from build123d import *

# Parameters (mm, degrees)
SKETCH1_R              = 1.5
SKETCH1_W              = 20
SKETCH1_H              = 1.5
SKETCH1_W_2            = 22.82
SKETCH1_H_2            = 7.086
BOSS_EXTRUDE1_DEPTH    = 5
SKETCH1_3_W            = 22.82
SKETCH1_3_H            = 1.114
BOSS_EXTRUDE2_DEPTH    = 1
CUT_EXTRUDE1_DEPTH     = 23.696190187
LPATTERN1_COUNT        = 4
LPATTERN1_PITCH        = 5
BOSS_EXTRUDE3_START    = -12
SKETCH1_5_W            = 22.82
SKETCH1_5_H            = 7.086
SKETCH1_5_H_2          = 1.114
BOSS_EXTRUDE3_DEPTH    = 12
SKETCH4_W              = 0.5
SKETCH4_H              = 0.5
BOSS_EXTRUDE4_DEPTH    = 5
SKETCH5_W              = 0.5
SKETCH5_H              = 2
BOSS_EXTRUDE5_DEPTH    = 8
FILLET1_R              = 1
LPATTERN2_COUNT        = 4
LPATTERN2_PITCH        = 5
FILLET1_OF_LPATTERN2_R = 1


with BuildPart() as part:
    # Sketch1 → Boss-Extrude1 (new body)
    # profile 1 of 3: a face of its own
    with BuildSketch(Plane.XY):
        Polygon((20, 7.493), (-20, 7.493), (-20, -7.493), (-11.41, -7.493), (-11.41, -0.407), (11.41, -0.407), (11.41, -7.493), (20, -7.493), align=None)
        with Locations((-15.24, 2.993)):
            Circle(SKETCH1_R, mode=Mode.SUBTRACT)
        with Locations((0, 1.743)):
            Rectangle(SKETCH1_W, SKETCH1_H, mode=Mode.SUBTRACT)
        with Locations((15.24, 2.993)):
            Circle(SKETCH1_R, mode=Mode.SUBTRACT)
    # profile 2 of 3: a face of its own
    with BuildSketch(Plane.XY):
        with Locations((0, -3.95)):
            Rectangle(SKETCH1_W_2, SKETCH1_H_2)
        with BuildLine():
            Line((-10, -0.607), (-5, -0.607))
            Line((-5, -0.607), (-5, -6.007))
            Line((-5, -6.007), (-5.9, -6.007))
            ThreePointArc((-5.9, -6.007), (-7.5, -6.807), (-9.1, -6.007))
            Line((-9.1, -6.007), (-10, -6.007))
            Line((-10, -6.007), (-10, -0.607))
        make_face(mode=Mode.SUBTRACT)
    # profile 3 of 3: a face of its own
    with BuildSketch(Plane.XY):
        with BuildLine():
            Line((-10, -6.007), (-9.1, -6.007))
            ThreePointArc((-9.1, -6.007), (-7.5, -6.807), (-5.9, -6.007))
            Line((-5.9, -6.007), (-5, -6.007))
            Line((-5, -6.007), (-5, -0.607))
            Line((-5, -0.607), (-10, -0.607))
            Line((-10, -0.607), (-10, -6.007))
        make_face()
    extrude(amount=BOSS_EXTRUDE1_DEPTH)

    # Sketch1<3> → Boss-Extrude2 (add)
    with BuildSketch(Plane.XY):
        Polygon((-11.41, -7.493), (-20, -7.493), (-20, -9.493), (20, -9.493), (20, -7.493), (11.41, -7.493), (11.41, -8.607), (-11.41, -8.607), align=None)
        with Locations((0, -8.05)):
            Rectangle(SKETCH1_3_W, SKETCH1_3_H)
    extrude(amount=BOSS_EXTRUDE2_DEPTH)

    # Sketch1<4> → Cut-Extrude1 (cut, through all)
    with BuildSketch(Plane.XY):
        with BuildLine():
            Line((-10, -6.007), (-9.1, -6.007))
            ThreePointArc((-9.1, -6.007), (-7.5, -6.807), (-5.9, -6.007))
            Line((-5.9, -6.007), (-5, -6.007))
            Line((-5, -6.007), (-5, -0.607))
            Line((-5, -0.607), (-10, -0.607))
            Line((-10, -0.607), (-10, -6.007))
        make_face()
    cut_extrude1 = extrude(amount=CUT_EXTRUDE1_DEPTH, mode=Mode.SUBTRACT)

    # LPattern1: Cut-Extrude1 ×4
    with Locations(*[(i * LPATTERN1_PITCH, 0, 0) for i in range(1, LPATTERN1_COUNT)]):
        add(cut_extrude1, mode=Mode.SUBTRACT)

    # Sketch1<5> → Boss-Extrude3 (add)
    # profile 1 of 3: a face of its own
    with BuildSketch(Plane.XY.offset(BOSS_EXTRUDE3_START)):
        with Locations((0, -3.95)):
            Rectangle(SKETCH1_5_W, SKETCH1_5_H)
        with BuildLine():
            Line((-10, -0.607), (-5, -0.607))
            Line((-5, -0.607), (-5, -6.007))
            Line((-5, -6.007), (-5.9, -6.007))
            ThreePointArc((-5.9, -6.007), (-7.5, -6.807), (-9.1, -6.007))
            Line((-9.1, -6.007), (-10, -6.007))
            Line((-10, -6.007), (-10, -0.607))
        make_face(mode=Mode.SUBTRACT)
    # profile 2 of 3: a face of its own
    with BuildSketch(Plane.XY.offset(BOSS_EXTRUDE3_START)):
        with BuildLine():
            Line((-10, -6.007), (-9.1, -6.007))
            ThreePointArc((-9.1, -6.007), (-7.5, -6.807), (-5.9, -6.007))
            Line((-5.9, -6.007), (-5, -6.007))
            Line((-5, -6.007), (-5, -0.607))
            Line((-5, -0.607), (-10, -0.607))
            Line((-10, -0.607), (-10, -6.007))
        make_face()
    # profile 3 of 3: a face of its own
    with BuildSketch(Plane.XY.offset(BOSS_EXTRUDE3_START)):
        with Locations((0, -8.05)):
            Rectangle(SKETCH1_5_W, SKETCH1_5_H_2)
    extrude(amount=BOSS_EXTRUDE3_DEPTH)

    # Sketch4 → Boss-Extrude4 (add)
    with BuildSketch(Plane.XY):
        with Locations((-7.5, -3.307)):
            Rectangle(SKETCH4_W, SKETCH4_H)
    boss_extrude4 = extrude(amount=BOSS_EXTRUDE4_DEPTH)

    # Sketch5 → Boss-Extrude5 (add)
    with BuildSketch(Plane(origin=(0, 0, -12), x_dir=(-1, 0, 0), z_dir=(0, 0, -1))):
        with Locations((8.245, -4.507)):
            Rectangle(SKETCH5_W, SKETCH5_H)
    boss_extrude5 = extrude(amount=BOSS_EXTRUDE5_DEPTH)

    # Fillet1
    fillet1_edges = [part.edges().sort_by_distance(p)[0] for p in [
        (-8.245, -5.507, -20),
        (-8.245, -3.507, -20),
    ]]
    fillet(fillet1_edges, radius=FILLET1_R - 0.0001)  # a hair under: the kernel refuses the full size

    # LPattern2: Boss-Extrude4, Boss-Extrude5 ×4
    with Locations(*[(i * LPATTERN2_PITCH, 0, 0) for i in range(1, LPATTERN2_COUNT)]):
        add(boss_extrude4)
        add(boss_extrude5)

    # Fillet1 of LPattern2
    fillet1_of_lpattern2_edges = [part.edges().sort_by_distance(p)[0] for p in [
        (-3.245, -5.507, -20),
        (-3.245, -3.507, -20),
        (1.755, -5.507, -20),
        (1.755, -3.507, -20),
        (6.755, -5.507, -20),
        (6.755, -3.507, -20),
    ]]
    fillet(fillet1_of_lpattern2_edges, radius=FILLET1_OF_LPATTERN2_R - 0.0001)  # a hair under: the kernel refuses the full size


solid = part.part
CAD build for the part. Positions are in the model's coordinates, mm. A direction names the side the tool comes from. Coordinates: 2 decimals unless noted, no trailing zeros. Order: outer loops, then holes, each group sorted by start corner. A loop starts at its lowest first (then second) coordinate and runs counter-clockwise, first axis right, second up.
Item 1: Band-saw the part on B-B on x = 15.24. List the corners of the cut face in (y, z).
Check sheet entries:
outline: (-9.49, 0) - (1.49, 0) - (1.49, 5) - (-7.49, 5) - (-7.49, 1) - (-9.49, 1) - close; (4.49, 0) - (7.49, 0) - (7.49, 5) - (4.49, 5) - close
Item 2: Two-plate mould, pull along Y, no slides. Class faces 6 (the face through (0, -4, -12)), 7 (the face through (-16.74, 3.06, 2.46)), 8 (the face through (-9.6, -6.007, 2.5)), 9 (the face through (0, -7.493, 3)): +Y half, -Y half, draft (parallel to the pull), parting line (faces both ways), or undercut.
Check sheet entries:
face 6: draft
face 7: undercut
face 8: undercut
face 9: -Y half
Item 3: Pin check, flat tips, straight feed: pin 1 Ø2 at (y, z) = (-5, -15) entering from +X (3 decimals); pin 2 Ø0.6 at (x, z) = (-8.5, -15.5) entering from -Y; pin 3 Ø1 at (x, y) = (-15.5, -6) entering from -Z. Stop position of each tip, or through.
Check sheet entries:
pin 1: stops at x = 7.005
pin 2: stops at y = -5.51
pin 3: stops at z = 0
Item 4: Band-saw the part on D-D on y = 2. List the corners of the cut face in (x, z).
Check sheet entries:
outline: (-20, 0) - (-16.36, 0) - (-16.36, 5) - (-20, 5) - close; (-14.12, 0) - (-10, 0) - (-10, 5) - (-14.12, 5) - close; (10, 0) - (14.12, 0) - (14.12, 5) - (10, 5) - close; (16.36, 0) - (20, 0) - (20, 5) - (16.36, 5) - close
Item 5: Drill centre lines: L1, parallel to X at y = -4.25, z = 0.25; L2, parallel to Y at x = -15.24, z = 3.45; L3, parallel to Z at x = -7, y = -6.5. Where is each one in solid material? Low to high.
Check sheet entries:
L1: x = -20 to -10, 10 to 20
L2: y = -7.49 to 1.49, 4.49 to 7.49
L3: z = -12 to 0
Item 6: Band-saw the part on C-C on y = -1.25. List the corners of the cut face in (x, z).
Check sheet entries:
outline: (-20, 0) - (-11.41, 0) - (-11.41, -12) - (11.41, -12) - (11.41, 0) - (20, 0) - (20, 5) - (10, 5) - (10, 0) - (-10, 0) - (-10, 5) - (-20, 5) - close
Item 7: Band-saw the part on A-A on z = -13. List the corners of the cut face in (x, y) (3 decimals).
Check sheet entries:
outline: (-8.495, -5.507) - (-7.995, -5.507) - (-7.995, -3.507) - (-8.495, -3.507) - close; (-3.495, -5.507) - (-2.995, -5.507) - (-2.995, -3.507) - (-3.495, -3.507) - close; (1.505, -5.507) - (2.005, -5.507) - (2.005, -3.507) - (1.505, -3.507) - close; (6.505, -5.507) - (7.005, -5.507) - (7.005, -3.507) - (6.505, -3.507) - close
Item 8: 3-axis set-ups, long thin cutter, end or side, ignore diameter. For faces 1 (the face through (0, 0.993, 2)), 2 (the face through (-7.526, -6.807, 2.465)), 3 (the face through (-7.995, -5, -16)), 4 (the face through (6.752, -3.792, -19.699)), 5 (the face through (-8.25, -5.22, -19.7)): which of +Z, -Z, +X, -X, +Y, -Y reach the whole face in a straight line?
Check sheet entries:
face 1: +Z, -Z
face 2: +Z
face 3: -Z, +Y, -Y
face 4: -Z, +X, -X, +Y
face 5: -Z, +X, -X, -Y
